Drawing for the job (mm, zero at the part's lowest x, y, z). A direction names the side the tool comes from. Coordinates: 2 decimals unless noted, no trailing zeros. Write each loop counter-clockwise with the first axis right and the second up, starting at its lowest first coordinate (ties: lowest second). Pieces come first, ordered by that corner, then holes. Notation, with made-up numbers: (-31.75, -12) -> (-23.75, -12) arc R26 ccw to (-23.75, 11) -> close; hole circle Ø10 at (63, -24.5). An arc over 180 degrees is marked (long way). Answer as CSV lines item,"result". Start each with the question number.
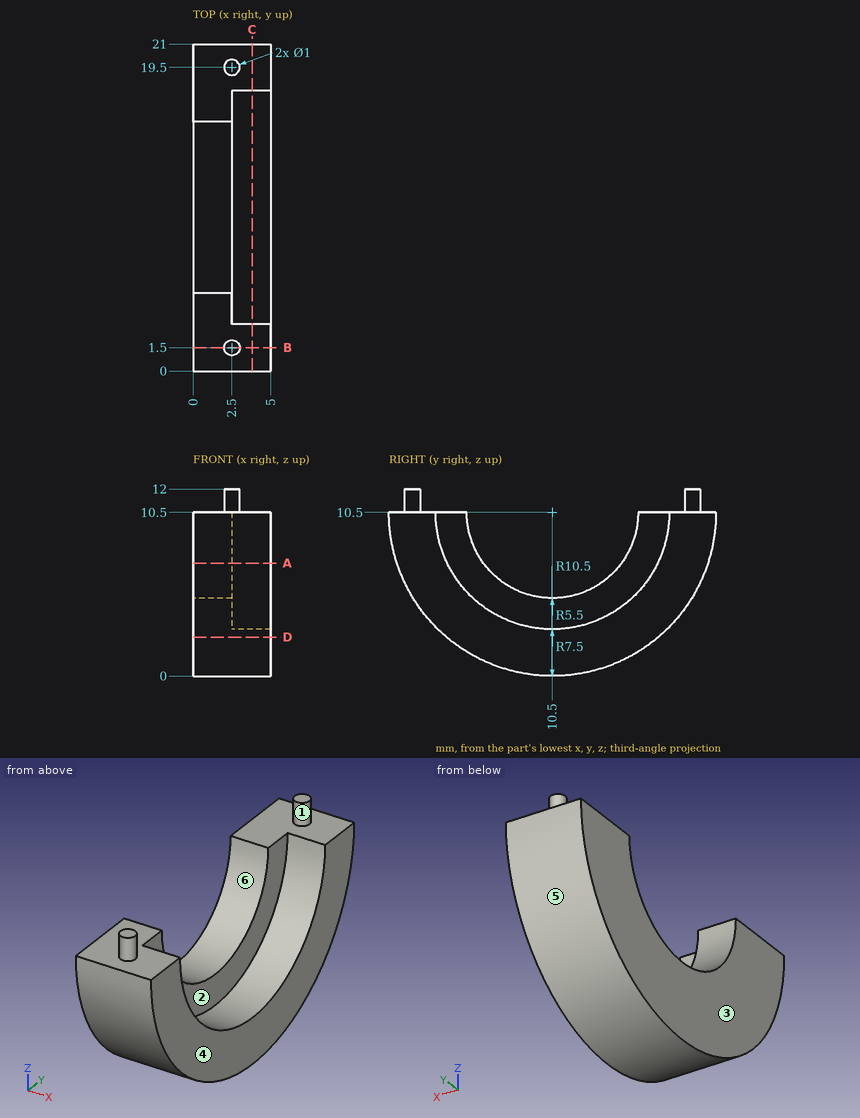
1. Cut at B-B (y = 1.5). Give the cut face in (x, z).
2. Wall check: line 1 (Z direction, x = 1.2, y = 10.5); line 2 (X direction, y = 4.5, z = 8.25); line 3 (Y direction, x = 1.85, z = 7.25). Give the ranges that are in metal, low to high.
3. Cut at A-A (z = 7.25). Give the cut face in (x, y), then the cut area to 3 significant figures.
4. Mould opens along Y. For the marked faces 4, 5 and 6 say: pulls with the +Y half, pulls with the -Y half, needs draft (parallel to the pull), parting line crosses it, or undercut.
5. Flat gauge pin, fed straight in: P1, Ø3, axis at x = 3.5, z = 7.5, coming from the +Y side. Where does the tip first touch, or does it go through?
6. Cut at D-D (z = 2.5). Give the cut face in (x, y).
7. Cut at C-C (x = 3.8). Give the cut face in (y, z).
8. Tool access for the marked faces 1, 2 and 3: list every direction of +Z, -Z, +X, -X, +Y, -Y with a clear straight run to the whole face (end or side of a thin tool).
Geometry check:
1,outline,"(0, 5.09) -> (5, 5.09) -> (5, 10.5) -> (3, 10.5) -> (3, 12) -> (2, 12) -> (2, 10.5) -> (0, 10.5) -> close"
2,line 1,"0 to 5"
2,line 2,"0 to 2.5"
2,line 3,"0.52 to 6.06, 14.94 to 20.48"
3,outline,"(0, 0.52) -> (5, 0.52) -> (5, 3.74) -> (2.5, 3.74) -> (2.5, 6.06) -> (0, 6.06) -> close; (0, 14.94) -> (2.5, 14.94) -> (2.5, 17.26) -> (5, 17.26) -> (5, 20.48) -> (0, 20.48) -> close"
3,area,"43.9 mm²"
4,face 4,"needs draft"
4,face 5,"parting line crosses it"
4,face 6,"undercut"
5,P1,"y = 20.89"
6,outline,"(0, 3.7) -> (5, 3.7) -> (5, 17.3) -> (0, 17.3) -> close"
7,outline,"(0, 10.5) arc R10.5 ccw to (21, 10.5) -> (18, 10.5) arc R7.5 cw to (3, 10.5) -> close"
8,face 1,"+Z"
8,face 2,"+Z, +X"
8,face 3,"+Z, -Z, -X, +Y, -Y"
